from build123d import *

# Parameters (mm, degrees)
RECTANGLE001_W       = 13
RECTANGLE001_H       = 22
PAD_DEPTH            = 12
RECTANGLE_FACE1_W    = 46
RECTANGLE_FACE1_H    = 22
PAD001_DEPTH         = 4
RECTANGLE002_FACE1_W = 22
RECTANGLE002_FACE1_H = 30
PAD002_DEPTH         = 4
RECTANGLE003_FACE1_W = 22
RECTANGLE003_FACE1_H = 13
PAD003_DEPTH         = 12
CIRCLE_R             = 3
POCKET_DEPTH         = 6
CIRCLE001_R          = 2.2
POCKET001_DEPTH      = 5
CIRCLE002_R          = 2.2
POCKET002_DEPTH      = 5
POCKET003_DEPTH      = 22
POCKET004_DEPTH      = 22
CHAMFER_SIZE         = 2
CHAMFER001_SIZE      = 1.7
FILLET_R             = 1.5
FILLET_FACE44_W      = 19
FILLET_FACE44_H      = 10.5
PAD004_DEPTH         = 0.01
SKETCH_W             = 6.073538
SKETCH_H             = 9.65966
PAD005_DEPTH         = 5
FILLET002_R          = 1.5


with BuildPart() as part:
    # Rectangle001 → Pad (new body)
    with BuildSketch(Plane(origin=(33, 0, 0), x_dir=(1, 0, 0), z_dir=(0, 0, 1))):
        with Locations((6.5, 11)):
            Rectangle(RECTANGLE001_W, RECTANGLE001_H)
    extrude(amount=PAD_DEPTH)

    # Rectangle Face1 → Pad001 (add)
    with BuildSketch(Plane.XY):
        with Locations((23, 11)):
            Rectangle(RECTANGLE_FACE1_W, RECTANGLE_FACE1_H)
    extrude(amount=-PAD001_DEPTH)

    # Rectangle002 Face1 → Pad002 (add)
    with BuildSketch(Plane(origin=(0, -30, 0), x_dir=(1, 0, 0), z_dir=(0, 0, 1))):
        with Locations((11, 15)):
            Rectangle(RECTANGLE002_FACE1_W, RECTANGLE002_FACE1_H)
    extrude(amount=-PAD002_DEPTH)

    # Rectangle003 Face1 → Pad003 (add)
    with BuildSketch(Plane(origin=(0, -30, 0), x_dir=(1, 0, 0), z_dir=(0, 0, 1))):
        with Locations((11, 6.5)):
            Rectangle(RECTANGLE003_FACE1_W, RECTANGLE003_FACE1_H)
    extrude(amount=PAD003_DEPTH)

    # Circle → Pocket (cut)
    with BuildSketch(Plane(origin=(8, 14, 0), x_dir=(1, 0, 0), z_dir=(0, 0, 1))):
        Circle(CIRCLE_R)
    extrude(amount=-POCKET_DEPTH, mode=Mode.SUBTRACT)

    # Circle001 → Pocket001 (cut)
    with BuildSketch(Plane(origin=(39.5, 11, 0), x_dir=(1, 0, 0), z_dir=(0, 0, 1))):
        Circle(CIRCLE001_R)
    extrude(amount=-POCKET001_DEPTH, mode=Mode.SUBTRACT)

    # Circle002 → Pocket002 (cut)
    with BuildSketch(Plane(origin=(11, -23.5, 0), x_dir=(1, 0, 0), z_dir=(0, 0, 1))):
        Circle(CIRCLE002_R)
    extrude(amount=-POCKET002_DEPTH, mode=Mode.SUBTRACT)

    # Circle002 → Pocket003 (cut)
    with BuildSketch(Plane(origin=(11, -23.5, 0), x_dir=(1, 0, 0), z_dir=(0, 0, 1))):
        Circle(CIRCLE002_R)
    extrude(amount=POCKET003_DEPTH, mode=Mode.SUBTRACT)

    # Circle001 → Pocket004 (cut)
    with BuildSketch(Plane(origin=(39.5, 11, 0), x_dir=(1, 0, 0), z_dir=(0, 0, 1))):
        Circle(CIRCLE001_R)
    extrude(amount=POCKET004_DEPTH, mode=Mode.SUBTRACT)

    # Chamfer
    chamfer_edges = [part.edges().sort_by_distance(p)[0] for p in [
        (5, 14, -4),
    ]]
    chamfer(chamfer_edges, length=CHAMFER_SIZE)

    # Chamfer001
    chamfer001_edges = [part.edges().sort_by_distance(p)[0] for p in [
        (8.8, -23.5, -4),
        (37.3, 11, -4),
    ]]
    chamfer(chamfer001_edges, length=CHAMFER001_SIZE)

    # Fillet
    fillet_edges = [part.edges().sort_by_distance(p)[0] for p in [
        (23, 22, -4),
        (0, -4, -4),
        (0, -17, 6),
        (0, -23.5, 12),
        (0, -30, 4),
        (11, -30, -4),
        (22, -15, -4),
        (34, 0, -4),
        (46, 11, -4),
        (11, -30, 12),
        (22, -23.5, 12),
        (22, -30, 4),
        (11, -17, 12),
        (22, -17, 6),
        (46, 11, 12),
        (33, 11, 12),
        (39.5, 0, 12),
        (46, 0, 4),
        (46, 22, 4),
        (33, 0, 6),
        (33, 22, 6),
        (39.5, 22, 12),
        (27.5, 0, 0),
        (22, -8.5, 0),
    ]]
    fillet(fillet_edges, radius=FILLET_R)

    # Fillet Face44 → Pad004 (add)
    with BuildSketch(Plane(origin=(33, 11, 5.25), x_dir=(0, 1, 0), z_dir=(-1, 0, 0))):
        Rectangle(FILLET_FACE44_W, FILLET_FACE44_H)
    extrude(amount=PAD004_DEPTH)

    # Sketch → Pad005 (join)
    with BuildSketch(Plane(origin=(33, -17, 0), x_dir=(-1, 0, 0), z_dir=(0, 1, 0))):
        with Locations((16.26208, 4.82983)):
            Rectangle(SKETCH_W, SKETCH_H)
    extrude(amount=PAD005_DEPTH)

    # Fillet002
    fillet002_edges = [part.edges().sort_by_distance(p)[0] for p in [
        (16.73792, -12, 9.65966),
        (19.774689, -12, 4.82983),
        (13.701151, -12, 4.82983),
        (13.701151, -14.5, 9.65966),
        (19.774689, -14.5, 9.65966),
    ]]
    fillet(fillet002_edges, radius=FILLET002_R)


solid = part.part
Part model, mm, in its own coordinate system. A direction names the side the tool comes from. Coordinates: 2 decimals unless noted, no trailing zeros. Order: outer loops, then holes, each group sorted by start corner. A loop starts at its lowest first (then second) coordinate and runs counter-clockwise, first axis right, second up.
(1) Slice it at A-A, the plane z = 3.75. State how many separate pieces and enclosed holes the cut face has, and give its area (3 significant figures).
Check sheet entries:
separate pieces: 2
enclosed holes: 2
area: 567 mm2
(2) Tool access for faces 4 (the face through (31.8, 22, -0.2)), 5 (the face through (19.347, -12.451, 4.137)), 6 (the face through (0.43, -17.45, 5.32)), 7 (the face through (32.99, 11, 5)): list every direction of +Z, -Z, +X, -X, +Y, -Y with a clear straight run to the whole face (end or side of a thin tool).
Check sheet entries:
face 4: +Z, -Z, +X, -X, +Y
face 5: +Z, +X, +Y
face 6: +Z, -X, +Y
face 7: +Z, -X, +Y, -Y
(3) Slice it at B-B, the plane x = 39.5. Write the cut outline in (y, z), and give its area (3 significant figures).
Check sheet entries:
outline: (0, -2.5) arc R1.5 ccw to (1.5, -4) - (7.1, -4) - (8.8, -2.3) - (8.8, 12) - (1.5, 12) arc R1.5 ccw to (0, 10.5) - close; (13.2, -2.3) - (14.9, -4) - (20.5, -4) arc R1.5 ccw to (22, -2.5) - (22, 10.5) arc R1.5 ccw to (20.5, 12) - (13.2, 12) - close
area: 277 mm2
(4) Probe L1, parallel to X at y = 11, z = 5.25; L2, parallel to X at y = -23.5, z = 3.5; L3, parallel to Y at x = 8, z = -0.75. List the from-to ranges inside material, lowest first.
Check sheet entries:
L1: x = 32.99 to 37.3, 41.7 to 46
L2: x = 0 to 8.8, 13.2 to 22
L3: y = -30 to 11, 17 to 22
(5) Slice it at D-D, the plane y = -4. Write the cut outline in (x, z).
Check sheet entries:
outline: (0, -2.5) arc R1.5 ccw to (1.5, -4) - (20.5, -4) arc R1.5 ccw to (22, -2.5) - (22, -1.5) arc R1.5 ccw to (20.5, 0) - (0, 0) - close
(6) Pin check, flat tips, straight feed: pin 1 Ø3 at (y, z) = (14.5, 4.5) entering from -X; pin 2 Ø1.5 at (x, y) = (23.5, 3.5) entering from +Z; pin 3 Ø3 at (y, z) = (-14.5, 5) entering from +X; pin 4 Ø8 at (x, z) = (22, 0.5) entering from -Y. Stop position of each tip, or through.
Check sheet entries:
pin 1: stops at x = 32.99
pin 2: stops at z = 0
pin 3: stops at x = 19.77
pin 4: stops at y = -30
(7) Pull direction Y, two halves, no side cores. Call faces 1 (the face through (17, -12, 4)), 2 (the face through (0.45, -3.6, -3.57)), 3 (the face through (10.523, -25.648, 4.95)): pulls with the +Y half, pulls with the -Y half, needs draft (parallel to the pull), parting line crosses it, or undercut.
Check sheet entries:
face 1: pulls with the +Y half
face 2: needs draft
face 3: undercut
